Verification items for the finished model (mm, model axes). A direction names the side the tool comes from. Coordinates: 2 decimals unless noted, no trailing zeros. Order: outer loops, then holes, each group sorted by start corner. A loop starts at its lowest first (then second) coordinate and runs counter-clockwise, first axis right, second up. Notation, with made-up numbers: (-11, 37.25) - (8, 37.25) arc R25 cw to (8, 76.25) - close; hole circle Ø1 at (72, 84.25). An arc over 180 degrees is marked (long way). Answer as CSV lines item,"result". Start each with the question number.
1. Set-up check for faces 1 (the flat face through (88, 0, 0)), 2 (the cylindrical face through (74.093, -0.867, 3.905)), 3 (the cylindrical face through (79.23, -1.08, 4.88)): record each of +Z, -Z, +X, -X, +Y, -Y from which the full face is reachable in a straight line by a thin tool's end or side.
2. Section check A-A (x = 19.5). Record the cut outline in (y, z).
3. Material ranges on L1, parallel to X at y = 3.5, z = 9.25; L2, parallel to Y at x = 81, z = 3; L3, parallel to X at y = 9, z = -11.75, recorded low to high. Write a range as [from, to].
4. Go/stop test with flat-tipped pins: pin 1 (8 mm diameter, centred on y = 1.5, z = -1, fed in from +X); pin 2 (8 mm diameter, centred on x = 52, z = -12, fed in from -Y); pin 3 (12 mm diameter, centred on x = 30.5, y = 3, fed in from +Z); pin 4 (5 mm diameter, centred on x = 49.5, z = -0.5, fed in from -Y). Record where each tip stops, or that it passes through.
Autodesk Inventor part; units mm, degrees
ref_plane "YZ Plane" through (0, 0, 0) normal (1, 0, 0) x (0, 1, 0)
ref_plane "XZ Plane" through (0, 0, 0) normal (0, 1, 0) x (-1, 0, 0)
ref_plane "XY Plane" through (0, 0, 0) normal (0, 0, 1) x (1, 0, 0)
sketch "Esboço1" plane through (0, 0, 0) normal (0, 0, 1) x (1, 0, 0)
  line L0 (0, 0) -> (88, 0)
  line L1 (88, 0) -> (88, 5)
  line L2 (88, 5) -> (3, 5)
  line L3 (3, 5) -> (3, 15)
  line L4 (3, 15) -> (0, 15)
  line L5 (0, 15) -> (0, 0)
  dimension "d0" = 88
  dimension "d1" = 5
  dimension "d2" = 3
  dimension "d3" = 15
revolve "Revolução1" add sketch "Esboço1" angle 360 about axis through (0, 0, 0) along (1, 0, 0)
chamfer "Chanfro1" distance 2 angle 45 1 edges at (3, -15, 0)
fillet "Arredondamento1" radius 4 1 edges at (88, -5, 0)
fillet "Arredondamento2" radius 1 1 edges at (3, -5, 0)
sketch "Esboço2" plane through (0, 0, 0) normal (0, 0, 1) x (1, 0, 0)
  line L0 (4, 5) -> (84, 5)
  line L1 (73.6, 5) -> (74.6, 5)
  line L2 (74.6, 5) -> (74.6, 4)
  line L3 (74.6, 4) -> (73.6, 4)
  line L4 (73.6, 4) -> (73.6, 5)
  line L5 (-17.6, 0) -> (105.6, 0)
  point P0 (0, 0)
  dimension "d10" = 1
  dimension "d11" = 4
  dimension "d12" = 73.6
revolve "Revolução2" cut sketch "Esboço2" angle 360 about axis through (-10, 0, 0) along (1, 0, 0)
Evaluation:
1,face 1,"+Z, -Z, +X, +Y, -Y"
1,face 2,"none"
1,face 3,"+X"
2,outline,"circle Ø10 at (0, 0)"
3,L1,"x = [0, 3]"
3,L2,"y = [-4, 4]"
3,L3,"x = [0, 1.2]"
4,pin 1,"stops at x = 88"
4,pin 2,"passes through"
4,pin 3,"stops at z = 5"
4,pin 4,"stops at y = -5"
